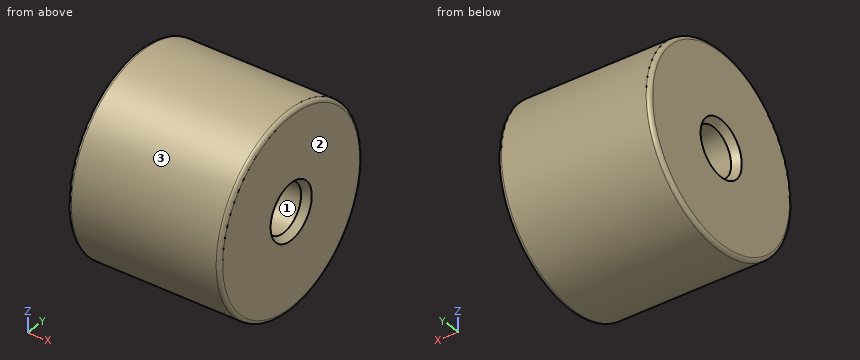
```python
from build123d import *

# Parameters (mm, degrees)
SKETCH1_W      = 30.48
SKETCH1_H      = 14.7295
CHAMFER1_SIZE  = 1.5
CHAMFER1_SIZE2 = 0.866025404
FILLET1_R      = 0.762
CHAMFER2_SIZE  = 1.5
CHAMFER2_SIZE2 = 0.866025404


with BuildPart() as part:
    # Sketch1 → Revolve1 (revolve)
    with BuildSketch(Plane.XY, mode=Mode.PRIVATE) as revolve1_sk:
        with Locations((0, 12.12975)):
            Rectangle(SKETCH1_W, SKETCH1_H)
    revolve(revolve1_sk.sketch.rotate(Axis((-1000, 0, 0), (1, 0, 0)), 90), axis=Axis((-1000, 0, 0), (1, 0, 0)))

    # Chamfer1
    chamfer1_edges = [part.edges().sort_by_distance(p)[0] for p in [
        (-15.24, 0, -4.765),
    ]]
    chamfer1_side = [part.faces().sort_by_distance(p)[0] for p in [
        (0, 0, -4.765),
    ]]
    chamfer(chamfer1_edges, length=CHAMFER1_SIZE, length2=CHAMFER1_SIZE2, reference=chamfer1_side[0])

    # Fillet1
    fillet1_edges = [part.edges().sort_by_distance(p)[0] for p in [
        (15.24, 0, -19.4945),
        (-15.24, 0, -19.4945),
    ]]
    fillet(fillet1_edges, radius=FILLET1_R)

    # Chamfer2
    chamfer2_edges = [part.edges().sort_by_distance(p)[0] for p in [
        (15.24, 0, -4.765),
    ]]
    chamfer2_side = [part.faces().sort_by_distance(p)[0] for p in [
        (0.75, 0, -4.765),
    ]]
    chamfer(chamfer2_edges, length=CHAMFER2_SIZE, length2=CHAMFER2_SIZE2, reference=chamfer2_side[0])


solid = part.part
```
Check sheet for the modelled part. Datum: model origin and axes. Units: mm. Face numbers are marked on the shaded views. Give positions to 0.01 mm unless a question says otherwise; leave off trailing zeros. Order: outer loops, then holes, each group sorted by start corner. A loop starts at its lowest first (then second) coordinate and runs counter-clockwise, first axis right, second up. Notation, with made-up numbers: (62, 7.5) -> (82, 7.5) arc R30 cw to (82, 41.5) -> close; hole circle Ø1 at (82.5, -39.5). An arc over 180 degrees is marked (long way). Use CSV: the item, a comma, the result in double quotes. Start each with the question number.
1) Go/stop test with flat-tipped pins: P1, Ø5, axis at x = 1, z = 3, coming from the -Y side; P2, Ø2, axis at x = 3.5, y = -9.5, coming from the -Z side; P3, Ø1, axis at x = -9, z = 12, coming from the -Y side. Record where each tip stops, or that it passes through.
2) Sectioned sample at A-A, the plane z = 0. Record the boundary of the cut face in (x, y) (1 decimal), plus the area to 3 significant figures.
3) Material ranges on line 1 (Y direction, x = -1, z = 0) (1 decimal); line 2 (Z direction, x = -9, y = -4); line 3 (Z direction, x = -5.5, y = -2.5), recorded low to high. Write a range as from..to.
4) Sectioned sample at C-C, the plane x = -9. Record the boundary of the cut face in (y, z) (1 decimal), plus the area to 3 significant figures.
5) Mould release check, pull along Y, two halves, no side actions. Record for the marked faces 1, 2 and 3: released by +Y, released by -Y, zero draft, split by the parting line, or undercut.
Recorded:
1,P1,"y = -19.49"
1,P2,"z = -17.54"
1,P3,"y = -15.74"
2,outline,"(-15.2, -18.7) arc R0.8 ccw to (-14.5, -19.5) -> (14.5, -19.5) arc R0.8 ccw to (15.2, -18.7) -> (15.2, -5.6) -> (13.7, -4.8) -> (-13.7, -4.8) -> (-15.2, -5.6) -> close; (-15.2, 5.6) -> (-13.7, 4.8) -> (13.7, 4.8) -> (15.2, 5.6) -> (15.2, 18.7) arc R0.8 ccw to (14.5, 19.5) -> (-14.5, 19.5) arc R0.8 ccw to (-15.2, 18.7) -> close"
2,area,"895 mm2"
3,line 1,"-19.5..-4.8, 4.8..19.5"
3,line 2,"-19.08..-2.59, 2.59..19.08"
3,line 3,"-19.33..-4.06, 4.06..19.33"
4,outline,"circle Ø39 at (0, 0); hole circle Ø9.5 at (0, 0)"
4,area,"1,120 mm2"
5,face 1,"undercut"
5,face 2,"zero draft"
5,face 3,"split by the parting line"
